Here's how the part is built. I have some questions about the finished solid (model axes, mm). A direction names the side the tool comes from. Coordinates: 2 decimals unless noted, no trailing zeros. Write each loop counter-clockwise with the first axis right and the second up, starting at its lowest first coordinate (ties: lowest second). Pieces come first, ordered by that corner, then holes. Notation, with made-up numbers: M 42.25,-40 L 85.25,-40 A33 cw 85.25,-3 Z; hole C 4.5,13 d7. An arc over 180 degrees is marked long. Use one line per item in the form item = value. Start each with the question number.
1. Please list where these lines run through material, in increasing order: line 1 along Z through (x, y) = (-1, 2.75); line 2 along Z through (x, y) = (3, -0.5); line 3 along X through (y, z) = (3.25, 19.5). Write a range as [from, to].
2. Thinking about a two-plate mould opening in Y: for faces 1 (the face through (-0.937, 4.806, 22.127)), 2 (the face through (0, 3, 0)), 3 (the face through (-0.91, 1.34, 22.13)), 4 (the face through (2.94, 2.18, 9.89)), which applies, released by +Y, released by -Y, zero draft, split by the parting line, or undercut?
3. On a 3-axis mill with a long thin cutter (end or side, diameter ignored), from which of +Z, -Z, +X, -X, +Y, -Y can I reach the whole of each face in a straight line? I mean faces 5 (the face through (1.091, 1.358, 22.127)), 6 (the face through (3.3, 2, 20)), 7 (the face through (2.38, 7.52, 21.85)). Say none if no direction works.
4. I want a section at A-A, the plane z = 21.5. List the corners of the cut face in (x, y) for me.
5. I'm going to push flat-ended pins straight in: pin 1 Ø2 at (x, y) = (-4, 7) entering from -Z; pin 2 Ø4 at (x, z) = (-3.5, 3.5) entering from +Y; pin 3 Ø2 at (x, z) = (-1.5, 21.5) entering from +Y. Where does each tip first touch, or does it pass through?
6. I want a section at B-B, the plane z = 4. List the corners of the cut face in (x, y) for me, plus the area to 3 significant figures.
Autodesk Inventor part; units mm, degrees
ref_plane "YZ Plane" through (0, 0, 0) normal (1, 0, 0) x (0, 1, 0)
ref_plane "XZ Plane" through (0, 0, 0) normal (0, 1, 0) x (-1, 0, 0)
ref_plane "XY Plane" through (0, 0, 0) normal (0, 0, 1) x (1, 0, 0)
sketch "Sketch1" plane through (0, 0, 0) normal (0, 0, 1) x (1, 0, 0)
  circle A0 centre (0.077, 3.0817) radius 3
  dimension "Diameter" = 6
extrude "Extrusion1" add sketch "Sketch1" along normal blind 20
sketch "Sketch2" plane through (0.077, 3.0817, 20) normal (0, 0, 1) x (1, 0, 0)
  circle A0 centre (0, 0) radius 3
  circle A1 centre (0, 0) radius 5
  dimension "Head_Diameter" = 10
extrude "Extrusion2" add sketch "Sketch2" along normal blind 4 contours A0 | A1
sketch "Sketch3" plane through (0.077, 3.0817, 24) normal (0, 0, 1) x (1, 0, 0)
  circle A0 centre (0, 0) radius 5
  line L0 (0, -2.3094) -> (-2, -1.1547)
  line L1 (-2, -1.1547) -> (-2, 1.1547)
  line L2 (-2, 1.1547) -> (0, 2.3094)
  line L3 (0, 2.3094) -> (2, 1.1547)
  line L4 (2, 1.1547) -> (2, -1.1547)
  line L5 (2, -1.1547) -> (0, -2.3094)
  dimension "Hex_Key_Size" = 4
extrude "Extrusion3" cut sketch "Sketch3" against normal blind 3.8 contours L0 L1 L2 L3 L4 L5
thread "Thread1"
fillet "Fillet1" radius 0.2 1 edges at (-2.923, 3.0817, 20)
chamfer "Chamfer1" distance 0.25 angle 45 2 edges at (-4.923, 3.0817, 24) (-2.923, 3.0817, 0)
equation "\"d9\" = Thread_Length"
equation "\"d13\" = Chamfer"
equation "\"Thread_Length\" = 18"
properties part number "SCREW,LOW SOCKET HD M6x1x20MM" material "Purchased Component, Altered"
Answer list:
q1.line_1 = [0, 20.2]
q1.line_2 = [20, 24]
q1.line_3 = [-2.92, 3.07]
q2.face_1 = undercut
q2.face_2 = zero draft
q2.face_3 = undercut
q2.face_4 = split by the parting line
q3.face_5 = +Z
q3.face_6 = -Z
q3.face_7 = +Z, -Z
q4.outline = C 0.08,3.08 d10; hole M -1.92,1.93 L 0.08,0.77 L 2.08,1.93 L 2.08,4.24 L 0.08,5.39 L -1.92,4.24 Z
q5.pin_1 = 20
q5.pin_2 = 5.63
q5.pin_3 = 8.05
q6.outline = C 0.08,3.08 d6
q6.area = 28.3 mm²
